Can you work these out from the drawing? Everything is in mm from the part's minimum corner. A direction names the side the tool comes from. Round coordinates to 2 decimals unless told otherwise and drop trailing zeros. Loops run counter-clockwise (first coordinate to the right, second up) from the corner with the lowest first, then second, coordinate; pieces in that order, holes last. Notation, with made-up numbers: (-25.5, -3.5) -> (5.5, -3.5) arc R9 cw to (5.5, 13.5) -> close; hole circle Ø5 at (20, -27). An arc over 180 degrees is marked (long way). One line per item, written item: value.
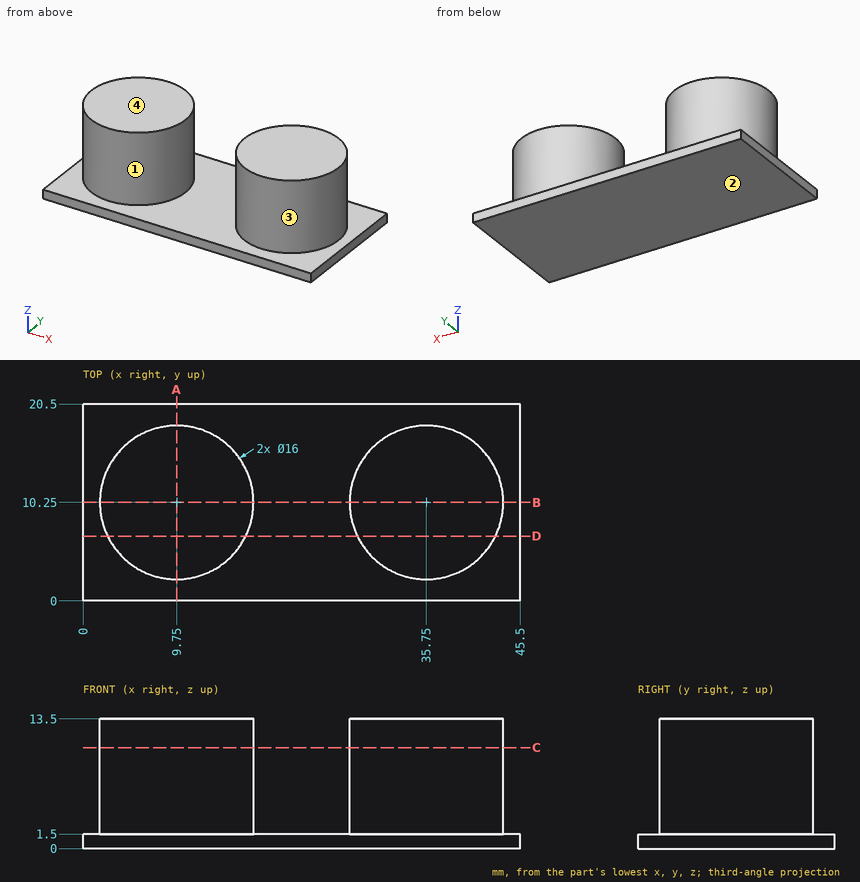
(1) If we section it at B-B, the plane y = 10.25: Please give me the cut outline in (x, z).
Recorded:
outline: (0, 0) -> (45.5, 0) -> (45.5, 1.5) -> (43.75, 1.5) -> (43.75, 13.5) -> (27.75, 13.5) -> (27.75, 1.5) -> (17.75, 1.5) -> (17.75, 13.5) -> (1.75, 13.5) -> (1.75, 1.5) -> (0, 1.5) -> close
(2) If I drill on L1, parallel to X at y = 10, z = 11; L2, parallel to Z at x = 19.5, y = 10.5; L3, parallel to X at y = 15.5, z = 11.75, over which ranges is the centre line in solid material (lowest first)?
Recorded:
L1: 1.75 to 17.75, 27.75 to 43.75
L2: 0 to 1.5
L3: 3.71 to 15.79, 29.71 to 41.79
(3) For the marked faces 1 and 2, which set-ups out of +Z, -Z, +X, -X, +Y, -Y let a thin tool reach every point of the face, with its end or its side?
Recorded:
face 1: +Z
face 2: -Z, +X, -X, +Y, -Y
(4) I'm going to push flat-ended pins straight in: pin 1 Ø2 at (x, z) = (16, 8) entering from -Y; pin 2 Ø1 at (y, z) = (3.5, 4) entering from +X; pin 3 Ø2 at (x, y) = (23.5, 10.5) entering from +Z; pin 4 Ø5 at (y, z) = (14.5, 2.5) entering from -X. Where does each tip first touch, or does it pass through?
Recorded:
pin 1: y = 4.21
pin 2: x = 40.74
pin 3: z = 1.5
pin 4: x = 0
(5) If we section it at C-C, the plane z = 10.5: Please give me the cut outline in (x, y).
Recorded:
outline: circle Ø16 at (9.75, 10.25); circle Ø16 at (35.75, 10.25)
(6) If we section it at D-D, the plane y = 6.75: Please give me the cut outline in (x, z).
Recorded:
outline: (0, 0) -> (45.5, 0) -> (45.5, 1.5) -> (42.94, 1.5) -> (42.94, 13.5) -> (28.56, 13.5) -> (28.56, 1.5) -> (16.94, 1.5) -> (16.94, 13.5) -> (2.56, 13.5) -> (2.56, 1.5) -> (0, 1.5) -> close
(7) Thinking about a two-plate mould opening in X: for the marked faces 3 and 4, which applies, released by +X, released by -X, zero draft, split by the parting line, or undercut?
Recorded:
face 3: undercut
face 4: zero draft
(8) If we section it at A-A, the plane x = 9.75: Please give me the cut outline in (y, z), then the cut area to 3 significant figures.
Recorded:
outline: (0, 0) -> (20.5, 0) -> (20.5, 1.5) -> (18.25, 1.5) -> (18.25, 13.5) -> (2.25, 13.5) -> (2.25, 1.5) -> (0, 1.5) -> close
area: 223 mm²
